Check sheet for the modelled part. Datum: model origin and axes. Units: mm. Face numbers are marked on the shaded views. A direction names the side the tool comes from. Coordinates: 2 decimals unless noted, no trailing zeros. Loops run counter-clockwise (first coordinate to the right, second up) from the corner with the lowest first, then second, coordinate; pieces in that order, holes last.
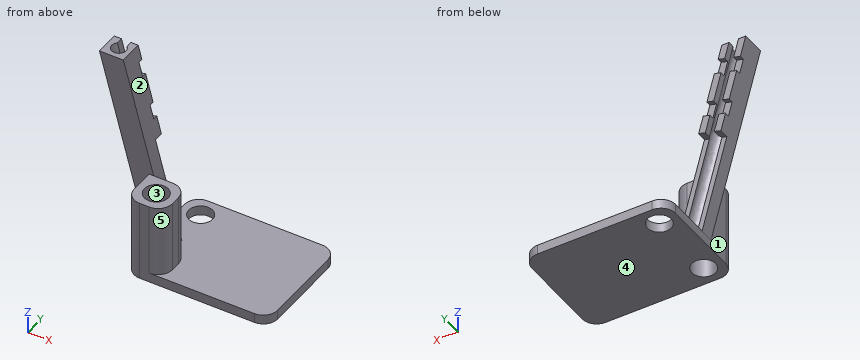
```python
from build123d import *

# Parameters (mm, degrees)
CROQUIS3_W              = 30
CROQUIS3_H              = 23
CROQUIS3_R              = 2.5
SALIENTE_EXTRUIR2_DEPTH = 2
CROQUIS5_W              = 8
CROQUIS5_H              = 8
CROQUIS5_R              = 2.5
SALIENTE_EXTRUIR3_DEPTH = 15
SALIENTE_EXTRUIR4_DEPTH = 40
REDONDEO1_R             = 3
CORTAR_EXTRUIR2_DEPTH   = 2
CORTAR_EXTRUIR3_DEPTH   = 1


with BuildPart() as part:
    # Croquis3 → Saliente-Extruir2 (new body)
    with BuildSketch(Plane.XY):
        with Locations((-48.169014085, 19.436619718)):
            Rectangle(CROQUIS3_W, CROQUIS3_H)
        with Locations((-59.169014085, 26.936619718)):
            Circle(CROQUIS3_R, mode=Mode.SUBTRACT)
        with Locations(Location((-59.169014085, 11.936619718, 0), (0, 0, 180))):
            Circle(CROQUIS3_R, mode=Mode.SUBTRACT)
    extrude(amount=SALIENTE_EXTRUIR2_DEPTH)

    # Croquis5 → Saliente-Extruir3 (add)
    with BuildSketch(Plane.XY.offset(2)):
        with Locations((-59.169014085, 11.936619718)):
            Rectangle(CROQUIS5_W, CROQUIS5_H)
        with Locations(Location((-59.169014085, 11.936619718, 0), (0, 0, 180))):
            Circle(CROQUIS5_R, mode=Mode.SUBTRACT)
    extrude(amount=SALIENTE_EXTRUIR3_DEPTH)

    # Croquis6 → Saliente-Extruir4 (add, along a direction that is not the sketch's normal)
    with BuildSketch(Plane.XY.offset(2)):
        with BuildLine():
            Line((-63.169014085, 15.936619718), (-58.169014085, 15.936619718))
            Line((-58.169014085, 15.936619718), (-58.169014085, 20.936619718))
            Line((-58.169014085, 20.936619718), (-59.669014085, 20.936619718))
            Line((-59.669014085, 20.936619718), (-59.669014085, 19.554653707))
            ThreePointArc((-59.669014085, 19.554653707), (-60.669014085, 16.936619718), (-61.669014085, 19.554653707))
            Line((-61.669014085, 19.554653707), (-61.669014085, 20.936619718))
            Line((-61.669014085, 20.936619718), (-63.169014085, 20.936619718))
            Line((-63.169014085, 20.936619718), (-63.169014085, 15.936619718))
        make_face()
    extrude(amount=SALIENTE_EXTRUIR4_DEPTH, dir=(-0.2588190451025139, 0, 0.9659258262890701))

    # Redondeo1
    redondeo1_edges = [part.edges().sort_by_distance(p)[0] for p in [
        (-33.169014085, 7.936619718, 1),
        (-33.169014085, 30.936619718, 1),
        (-63.169014085, 7.936619718, 8.5),
        (-63.169014085, 30.936619718, 1),
        (-55.169014085, 7.936619718, 9.5),
        (-55.169014085, 15.936619718, 9.5),
    ]]
    fillet(redondeo1_edges, radius=REDONDEO1_R)

    # Croquis10 → Cortar-Extruir2 (cut)
    with BuildSketch(Plane(origin=(0, 20.936619718, 0), x_dir=(1, 0, 0), z_dir=(0, 1, 0))):
        Polygon((-58.169014085, -2), (-63.169014085, -2), (-68.345394987, -21.318516526), (-63.680331477, -22.568516526), align=None)
    extrude(amount=-CORTAR_EXTRUIR2_DEPTH, mode=Mode.SUBTRACT)

    # Croquis11 → Cortar-Extruir3 (cut)
    with BuildSketch(Plane(origin=(0, 20.936619718, 0), x_dir=(1, 0, 0), z_dir=(0, 1, 0))):
        Polygon((-64.639490212, -26.148145657), (-69.304553722, -24.898145657), (-70.081010857, -27.795923136), (-65.415947347, -29.045923136), align=None)
        Polygon((-66.968861618, -34.841478094), (-71.633925127, -33.591478094), (-72.410382263, -36.489255573), (-67.745318753, -37.739255573), align=None)
    extrude(amount=-CORTAR_EXTRUIR3_DEPTH, mode=Mode.SUBTRACT)


solid = part.part
```
1) Set-up check for the marked faces 4 and 5: record each of +Z, -Z, +X, -X, +Y, -Y from which the full face is reachable in a straight line by a thin tool's end or side.
Answer sheet:
face 4: -Z, +X, -X, +Y, -Y
face 5: +Z, +X, -Y
2) Mould release check, pull along X, two halves, no side actions. Record for the marked faces 1, 2 and 3: +X half, -X half, draft (parallel to the pull), parting line (faces both ways), or undercut.
Answer sheet:
face 1: -X half
face 2: +X half
face 3: undercut
3) Depth check by flat-ended pin: pin 1 (4.5 mm diameter, centred on x = -59.5, z = 10, fed in from +Y); pin 2 (2.5 mm diameter, centred on x = -67.5, z = 35.5, fed in from +Y); pin 3 (0.6 mm diameter, centred on y = 12, z = 7.5, fed in from +X); pin 4 (3 mm diameter, centred on x = -59.17, y = 11.94, fed in from +Z). Enter the tip coordinate at first touch or a pass-through.
Answer sheet:
pin 1: stops at y = 18.94
pin 2: stops at y = 20.94
pin 3: stops at x = -55.17
pin 4: passes through
4) Scan lines: line 1 (Z direction, x = -45, y = 23); line 2 (X direction, y = 18.75, z = 36.5); line 3 (X direction, y = 17.5, z = 32.5). Record each from-to range of solid material in increasing order.
Answer sheet:
line 1: z = 0 to 2
line 2: x = -72.41 to -71.38, -68.45 to -67.41
line 3: x = -71.34 to -70.01, -67.67 to -66.34
5) Section check A-A on x = -49.5. Enter the section's corners in (y, z), plus the area to 3 significant figures.
Answer sheet:
outline: (7.94, 0) - (30.94, 0) - (30.94, 2) - (7.94, 2) - close
area: 46.0 mm2
